```python
from build123d import *

# Parameters (mm, degrees)
SKETCH1_W           = 560
SKETCH1_H           = 60
BOSS_EXTRUDE1_DEPTH = 10
SKETCH2_W           = 10
SKETCH2_H           = 60
BOSS_EXTRUDE2_DEPTH = 45
SKETCH3_R           = 11
SKETCH3_R_2         = 4
CUT_EXTRUDE1_DEPTH  = 440
SKETCH4_R           = 5
BOSS_EXTRUDE3_DEPTH = 10


with BuildPart() as part:
    # Sketch1 → Boss-Extrude1 (new body)
    with BuildSketch(Plane(origin=(0, 0, 0), x_dir=(1, 0, 0), z_dir=(0, 1, 0))):
        Rectangle(SKETCH1_W, SKETCH1_H)
    extrude(amount=BOSS_EXTRUDE1_DEPTH)

    # Sketch2 → Boss-Extrude2 (add)
    with BuildSketch(Plane(origin=(0, 10, 0), x_dir=(1, 0, 0), z_dir=(0, 1, 0))):
        with Locations((-175, 0)):
            Rectangle(SKETCH2_W, SKETCH2_H)
        with Locations((250, 0)):
            Rectangle(SKETCH2_W, SKETCH2_H)
    extrude(amount=BOSS_EXTRUDE2_DEPTH)

    # Sketch3 → Cut-Extrude1 (cut)
    with BuildSketch(Plane.ZY.offset(180)):
        with Locations((-8.85, 31.15)):
            Circle(SKETCH3_R)
        with Locations((21.15, 31.15)):
            Circle(SKETCH3_R_2)
    extrude(amount=-CUT_EXTRUDE1_DEPTH, mode=Mode.SUBTRACT)

    # Sketch4 → Boss-Extrude3 (add)
    with BuildSketch(Plane.XZ):
        with Locations(Location((-270, 0, 0), (0, 0, 90))):
            Circle(SKETCH4_R)
        with Locations(Location((260, 0, 0), (0, 0, 90))):
            Circle(SKETCH4_R)
    extrude(amount=BOSS_EXTRUDE3_DEPTH)


solid = part.part
```
Verification items for the finished model (mm, model axes). A direction names the side the tool comes from. Coordinates: 2 decimals unless noted, no trailing zeros. Loops run counter-clockwise (first coordinate to the right, second up) from the corner with the lowest first, then second, coordinate; pieces in that order, holes last. Notation, with made-up numbers: (76.25, -10) -> (134.25, -10) arc R21 cw to (134.25, 3) -> close; hole circle Ø7 at (16, -2). An arc over 180 degrees is marked (long way). Answer in a Markdown table with one row per item.
1) Section check A-A (x = -270). Record the cut outline in (y, z), and give its area (3 significant figures).
The answers:
| item | result |
|---|---|
| outline | (-10, -5) -> (0, -5) -> (0, -30) -> (10, -30) -> (10, 30) -> (0, 30) -> (0, 5) -> (-10, 5) -> close |
| area | 700 mm2 |
2) Section check B-B (x = -150.5). Record the cut outline in (y, z), and give its area (3 significant figures).
The answers:
| item | result |
|---|---|
| outline | (0, -30) -> (10, -30) -> (10, 30) -> (0, 30) -> close |
| area | 600 mm2 |
3) Access from +Z, -Z, +X, -X, +Y, -Y to the whole of each face (thin tool, end or side, straight path). Record for faces 1 (the face through (-180, 32, 7)), 2 (the face through (255.043, -4.93, -0.651)), 3 (the face through (255, 32, 7)), 4 (the face through (-270, -10, 0)), 5 (the face through (-170, 32, 7)).
The answers:
| item | result |
|---|---|
| face 1 | +Z, -Z, -X, +Y |
| face 2 | -Y |
| face 3 | +Z, -Z, +X, +Y |
| face 4 | +Z, -Z, +X, -X, -Y |
| face 5 | +Z, -Z, +Y |
4) Draft check along Z on faces 6 (the face through (249.9, 40.4, -2.9)), 7 (the face through (-274.957, -4.93, -0.651)), 8 (the face through (280, 5, 0)). Enter one of: released by +Z, released by -Z, zero draft, split by the parting line, or undercut.
The answers:
| item | result |
|---|---|
| face 6 | undercut |
| face 7 | split by the parting line |
| face 8 | zero draft |
5) Scan lines: line 1 along Y through (x, z) = (248.5, -8.85); line 2 along X through (y, z) = (21, -4.5); line 3 along Y through (x, z) = (250.75, 21.15). Record each from-to range of solid material in increasing order. Write a range as from..to.
The answers:
| item | result |
|---|---|
| line 1 | y = 0..20.15, 42.15..55 |
| line 2 | x = -180..-170, 245..255 |
| line 3 | y = 0..27.15, 35.15..55 |
6) Depth check by flat-ended pin: P1, Ø10, axis at y = 42, z = 14.5, coming from the +X side; P2, Ø13.5, axis at y = 21.5, z = 10, coming from the -X side; P3, Ø18, axis at x = -253.5, z = 7.5, coming from the +Y side; P4, Ø6.5, axis at y = 31.15, z = 21.15, coming from the -X side. Enter the tip coordinate at first touch or a pass-through.
The answers:
| item | result |
|---|---|
| P1 | stops at x = 255 |
| P2 | stops at x = -180 |
| P3 | stops at y = 10 |
| P4 | passes through |
